Design review of the part built by this model. Coordinates are the model's own, in mm. Face numbers are marked on the shaded views. A direction names the side the tool comes from. Coordinates: 2 decimals unless noted, no trailing zeros. Order: outer loops, then holes, each group sorted by start corner. A loop starts at its lowest first (then second) coordinate and runs counter-clockwise, first axis right, second up. Notation, with made-up numbers: M -23.75,-6.75 L -17.75,-6.75 A31 ccw -17.75,27.25 Z; hole C -36.75,11.5 d9. An arc over 180 degrees is marked long. Use CSV: the item, a comma, the result in double quotes.
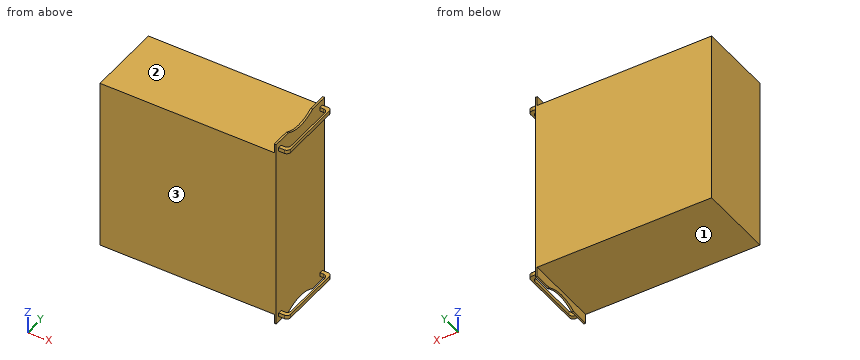
Autodesk Inventor part; units mm, degrees
ref_plane "YZ Plane" through (0, 0, 0) normal (1, 0, 0) x (0, 1, 0)
ref_plane "XZ Plane" through (0, 0, 0) normal (0, 1, 0) x (-1, 0, 0)
ref_plane "XY Plane" through (0, 0, 0) normal (0, 0, 1) x (1, 0, 0)
sketch "Sketch1" plane through (0, 0, 0) normal (0, 1, 0) x (-1, 0, 0)
  line L0 (232.5, 230) -> (-232.5, 230)
  line L1 (-232.5, 230) -> (-232.5, -230)
  line L2 (-232.5, -230) -> (232.5, -230)
  line L3 (232.5, -230) -> (232.5, 230)
  line L4 (232.5, 230) -> (-232.5, -230) construction
  line L5 (-232.5, 230) -> (232.5, -230) construction
  point P0 (0, 0)
  dimension "d0" = 465
  dimension "d1" = 460
extrude "Extrusion1" add sketch "Sketch1" along normal blind 200
sketch "Sketch3" plane through (232.5, 0, -230) normal (0, 0, -1) x (-1, 0, 0)
  line L0 (0, 0) -> (0, 200)
  line L1 (0, 200) -> (5, 200)
  line L2 (0, 200) -> (465, 200)
  line L3 (5, 200) -> (5, 0)
  line L4 (5, 0) -> (0, 0)
  line L5 (0, 0) -> (0, 200)
  point P0 (232.5, 0)
  dimension "d6" = 5
extrude "Extrusion3" add sketch "Sketch3" along normal blind 25
sketch "Sketch4" plane through (-232.5, 0, 230) normal (0, 0, 1) x (1, 0, 0)
  line L0 (465, 0) -> (465, 200)
  line L1 (465, 200) -> (465, 0)
  line L2 (465, 0) -> (460, 0)
  line L3 (0, 0) -> (465, 0)
  line L4 (460, 0) -> (460, 200)
  line L5 (0, 200) -> (465, 200)
  point P0 (232.5, 0)
  dimension "d10" = 5
extrude "Extrusion4" add sketch "Sketch4" along normal blind 25
sketch "Sketch5" plane through (232.5, 0, -255) normal (1, 0, 0) x (0, 0, -1)
  line L0 (-510, 100) -> (0, 100)
  line L1 (0, 200) -> (0, 0)
  line L2 (-510, 100) -> (-510, 150)
  line L3 (-510, 0) -> (-510, 200)
  line L4 (-510, 100) -> (-510, 50)
  line L5 (-510, 100) -> (-460, 100) construction
  arc A0 (-510, 50) -> (-510, 150) centre (-596.6025, 100) ccw
  line L6 (0, 100) -> (0, 150)
  line L7 (0, 100) -> (0, 50)
  arc A1 (0, 150) -> (0, 50) centre (86.6025, 100) ccw
  point P0 (-255, 0)
  point P1 (-510, 50)
  dimension "d13" = 50
  dimension "d14" = 50
  dimension "d15" = 90
  dimension "d16" = 100
  dimension "d17" = 50
  dimension "d18" = 100
extrude "Extrusion5" cut sketch "Sketch5" against normal blind 25
sketch "Sketch6" plane through (232.5, 0, 255) normal (1, 0, 0) x (0, 0, -1)
  line L0 (25, 0) -> (25, 200)
  line L1 (25, 190) -> (25, 180)
  line L2 (25, 180) -> (15, 180)
  line L3 (15, 180) -> (15, 190)
  line L4 (15, 190) -> (25, 190)
  point P0 (255, 0)
  point P1 (0, 200)
  dimension "d22" = 10
  dimension "d23" = 10
extrude "Extrusion6" add sketch "Sketch6" along normal blind 25
mirror "Mirror1" about plane through (0, 0, 0) normal (0, 0, 1) of "Extrusion6"
sketch "Sketch7" plane through (232.5, 0, 255) normal (1, 0, 0) x (0, 0, -1)
  line L0 (0, 0) -> (510, 0)
  line L1 (0, 50) -> (0, 0)
  line L2 (25, 0) -> (25, 200)
  line L3 (25, 10) -> (25, 20)
  line L4 (25, 20) -> (15, 20)
  line L5 (15, 20) -> (15, 10)
  line L6 (15, 10) -> (25, 10)
  point P0 (255, 0)
  dimension "d27" = 10
  dimension "d28" = 10
extrude "Extrusion7" add sketch "Sketch7" along normal blind 25
mirror "Mirror2" about plane through (0, 0, 0) normal (0, 0, 1) of "Extrusion7"
sketch "Sketch8" plane through (232.5, 20, 240) normal (0, 1, 0) x (1, 0, 0)
  line L0 (25, 10) -> (25, 0)
  line L1 (25, 0) -> (25, 10)
  line L2 (25, 10) -> (20, 10)
  line L3 (0, 10) -> (25, 10)
  line L4 (20, 10) -> (20, 0)
  line L5 (0, 0) -> (25, 0)
  line L6 (25, 0) -> (20, 0)
  point P0 (-232.5, 240)
  dimension "d31" = 5
  dimension "d32" = 90
extrude "Extrusion8" add sketch "Sketch8" along normal blind 160
mirror "Mirror3" about plane through (0, 0, 0) normal (0, 0, 1) of "Extrusion8"
fillet "Face Fillet1" radius 10 1 edges at (252.5, 20, 235)
fillet "Face Fillet2" radius 10 1 edges at (257.5, 10, 235)
fillet "Face Fillet3" radius 10 1 edges at (257.5, 10, -235)
fillet "Face Fillet4" radius 10 1 edges at (257.5, 190, -235)
fillet "Face Fillet5" radius 10 1 edges at (257.5, 190, 235)
fillet "Face Fillet6" radius 10 1 edges at (252.5, 20, -235)
fillet "Face Fillet7" radius 10 1 edges at (252.5, 180, -235)
fillet "Face Fillet8" radius 10 1 edges at (252.5, 180, 235)
properties part number "PC"
(1) Add section B-B on x = 66. State the section outline as (y, z) points, and give its area (3 significant figures).
The answers:
outline,"M 0,-230 L 200,-230 L 200,230 L 0,230 Z"
area,"92,000 mm2"
(2) Add section C-C on z = -176.5. State the section outline as (x, y) points.
The answers:
outline,"M -232.5,0 L 232.5,0 L 232.5,200 L -232.5,200 Z"
(3) Wall thickness on probe 1 along X at (y, z) = (45, 19); probe 2 along Z at (x, y) = (35, 121): over which ranges is each line inside the solid? List them lowest first.
The answers:
probe 1,"x = -232.5 to 232.5"
probe 2,"z = -230 to 230"
(4) For the marked faces 1, 2 and 3, list the 3-axis set-ups (+Z, -Z, +X, -X, +Y, -Y) from which the entire face can be reached by the end or side of a thin tool; tool diameter is ignored.
The answers:
face 1,"-Z, -X, +Y, -Y"
face 2,"+Z, -X, +Y, -Y"
face 3,"+Z, -Z, +X, -X, -Y"
(5) Clearance check with flat-ended pins moving along their axes: P1, Ø5, axis at x = 239.5, z = -233, coming from the +Y side; P2, Ø5, axis at x = 243.5, z = 233.5, coming from the -Y side; P3, Ø3, axis at y = 108.5, z = 236, coming from the -X side; P4, Ø12.5, axis at x = 239.5, y = 115.5, coming from the +Z side (3 decimals). State where each tip first meets the part, or that it passes through.
The answers:
P1,"stops at y = 190"
P2,"stops at y = 10"
P3,"stops at x = 227.5"
P4,"passes through"
(6) Add section D-D on y = 62.5. State the section outline as (x, z) points, and give its area (3 significant figures).
The answers:
outline,"M -232.5,-230 L 227.5,-230 L 227.5,-248.9 L 232.5,-248.9 L 232.5,248.9 L 227.5,248.9 L 227.5,230 L -232.5,230 Z; M 252.5,-240 L 257.5,-240 L 257.5,-230 L 252.5,-230 Z; M 252.5,230 L 257.5,230 L 257.5,240 L 252.5,240 Z"
area,"214,000 mm2"
(7) Add section A-A on y = 157. State the section outline as (x, z) points, and give its area (3 significant figures).
The answers:
outline,"M -232.5,-230 L 227.5,-230 L 227.5,-255 L 232.5,-255 L 232.5,255 L 227.5,255 L 227.5,230 L -232.5,230 Z; M 252.5,-240 L 257.5,-240 L 257.5,-230 L 252.5,-230 Z; M 252.5,230 L 257.5,230 L 257.5,240 L 252.5,240 Z"
area,"214,000 mm2"
